```python
from build123d import *

# Parameters (mm, degrees)
F0_R     = 17.526
F1_DEPTH = 2.54
F3_DEPTH = 8.89
F4_SIZE  = 0.762
F5_SIZE  = 0.508


with BuildPart() as f1:
    # F0 (on Top) → F1 (new body)
    with BuildSketch(Plane.XY):
        Circle(F0_R)
    extrude(amount=F1_DEPTH)

    # F2 (on face) → F3 (join)
    with BuildSketch(Plane.XY.offset(2.54)):
        with BuildLine():
            Line((8.76415, -12.7), (8.76415, 12.7))
            ThreePointArc((8.76415, 12.7), (-15.4305, 0), (8.76415, -12.7))
        make_face()
    extrude(amount=F3_DEPTH)

    # F4
    f4_edges = [f1.edges().sort_by_distance(p)[0] for p in [
        (-15.4305, 0, 11.43),
        (8.76415, 0, 11.43),
        (8.76415, 0, 2.54),
        (-15.4305, 0, 2.54),
    ]]
    chamfer(f4_edges, length=F4_SIZE)

    # F5
    f5_edges = [f1.edges().sort_by_distance(p)[0] for p in [
        (-17.526, 0, 2.54),
        (-17.526, 0, 0),
    ]]
    chamfer(f5_edges, length=F5_SIZE)


solid = f1.part
```
CAD build for the part. Positions are in the model's coordinates, mm. A direction names the side the tool comes from. Round coordinates to 2 decimals unless told otherwise and drop trailing zeros. Write each loop counter-clockwise with the first axis right and the second up, starting at its lowest first coordinate (ties: lowest second). Pieces come first, ordered by that corner, then holes. Notation, with made-up numbers: (33.5, -0.75) -> (41.5, -0.75) arc R32 ccw to (41.5, 26.25) -> close; hole circle Ø1 at (-35, 37). An arc over 180 degrees is marked (long way). Answer in a Markdown table with one row per item. Add a question column.
Item 1: Mould opens along Y. For faces 1 (the face through (8.764, 0, 7)), 2 (the face through (-15.545, 0.479, 3.18)) say: pulls with the +Y half, pulls with the -Y half, needs draft (parallel to the pull), parting line crosses it, or undercut.
Item 2: Which spindle directions (+Z, -Z, +X, -X, +Y, -Y) get a long thin tool onto all of the face, cutting with end or side? Do faces 3 (the face through (0, 0, 0)), 4 (the face through (-15.423, 0.47, 6.933)). Say none if no direction does.
Item 3: Drop flat-ended pins along their axis: pin 1 Ø6 at (y, z) = (12.5, 2) entering from -X; pin 2 Ø3 at (y, z) = (4, 1.5) entering from -X; pin 3 Ø6 at (x, z) = (4, 6.5) entering from +Y. Give the stop position or say it passes through.
Item 4: Saw through at C-C, the plane z = 7.75. Write the cut outline in (x, y).
Item 5: Drill centre lines: line 1 (Z direction, x = 14, y = -5.5); line 2 (X direction, y = 0.5, z = 0.75); line 3 (Y direction, x = 4, z = 9.25). Where is each one in solid material? Low to high. Write a range as from..to.
Item 6: Saw through at A-A, the plane x = 0. Write the cut outline in (y, z), then the cut area to 3 significant figures.
Item 7: Saw through at B-B, the plane y = 0. Write the cut outline in (x, z), then the cut area to 3 significant figures.
Findings below:
| question | item | result |
|---|---|---|
| 1 | face 1 | needs draft |
| 1 | face 2 | parting line crosses it |
| 2 | face 3 | -Z, +X, -X, +Y, -Y |
| 2 | face 4 | +Z |
| 3 | pin 1 | stops at x = -14.73 |
| 3 | pin 2 | stops at x = -17.35 |
| 3 | pin 3 | stops at y = 15.4 |
| 4 | outline | (8.76, -12.7) -> (8.76, 12.7) arc R15.43 ccw (long way) to start |
| 5 | line 1 | z = 0..2.54 |
| 5 | line 2 | x = -17.52..17.52 |
| 5 | line 3 | y = -14.9..14.9 |
| 6 | outline | (-17.53, 0.51) -> (-17.02, 0) -> (17.02, 0) -> (17.53, 0.51) -> (17.53, 2.03) -> (17.02, 2.54) -> (16.19, 2.54) -> (15.43, 3.3) -> (15.43, 10.67) -> (14.67, 11.43) -> (-14.67, 11.43) -> (-15.43, 10.67) -> (-15.43, 3.3) -> (-16.19, 2.54) -> (-17.02, 2.54) -> (-17.53, 2.03) -> close |
| 6 | area | 363 mm^2 |
| 7 | outline | (-17.53, 0.51) -> (-17.02, 0) -> (17.02, 0) -> (17.53, 0.51) -> (17.53, 2.03) -> (17.02, 2.54) -> (9.53, 2.54) -> (8.76, 3.3) -> (8.76, 10.67) -> (8, 11.43) -> (-14.67, 11.43) -> (-15.43, 10.67) -> (-15.43, 3.3) -> (-16.19, 2.54) -> (-17.02, 2.54) -> (-17.53, 2.03) -> close |
| 7 | area | 304 mm^2 |
